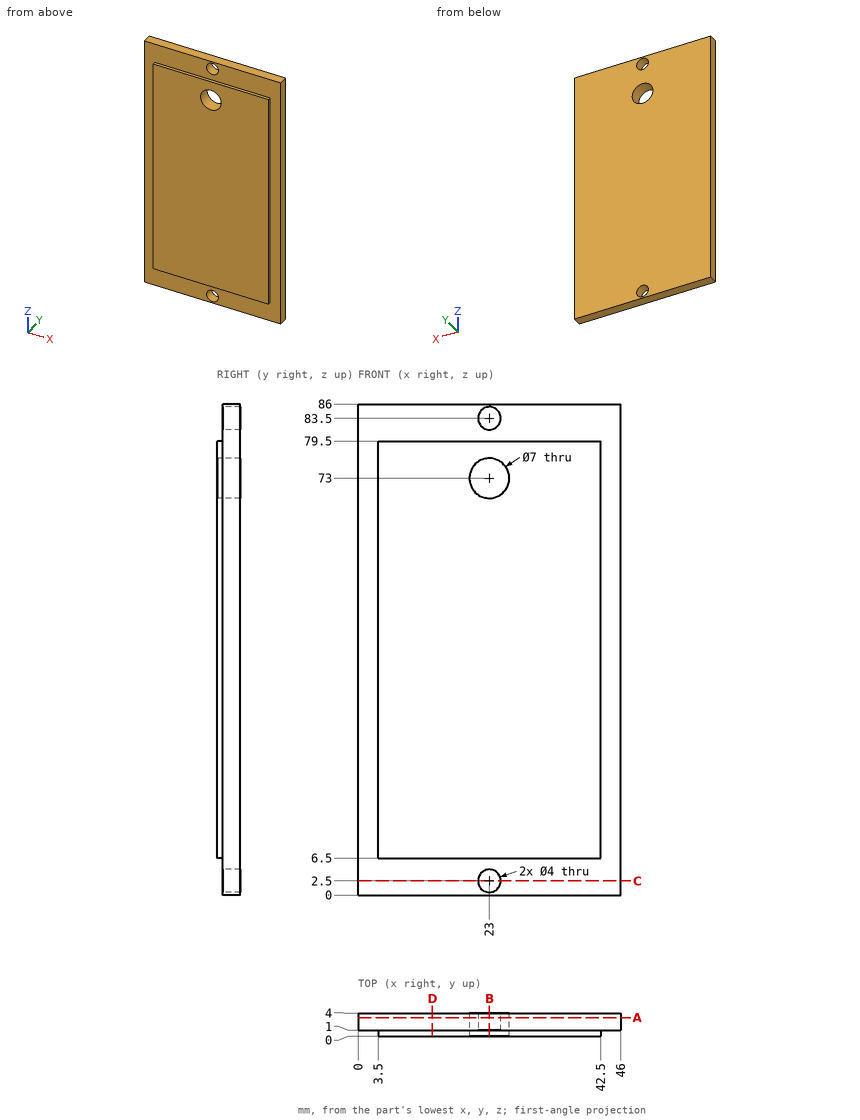
Job drawing, mm, ordinate dimensions from the low corner. One solid piece. Coordinates: 2 decimals unless noted, no trailing zeros. Order: outer loops, then holes, each group sorted by start corner. A loop starts at its lowest first (then second) coordinate and runs counter-clockwise, first axis right, second up. Notation, with made-up numbers: M 33,62 L 87,62 A30 ccw 87,86 Z; hole C 71.25,-30.5 d1. An arc over 180 degrees is marked long. Return JSON: item names as keys, results as strings.
1. Drill centre lines: probe 1 along Z at (x, y) = (23, 2.3); probe 2 along X at (y, z) = (2.5, 83.5); probe 3 along Z at (x, y) = (24.5, 3.1). Where is each one in solid material? Low to high.
Ans:
{"probe 1": "0 to 0.5, 4.5 to 69.5, 76.5 to 81.5, 85.5 to 86", "probe 2": "0 to 21, 25 to 46", "probe 3": "0 to 1.18, 3.82 to 69.84, 76.16 to 82.18, 84.82 to 86"}
2. Saw through at A-A (y = 3.2). Give the cut face in (x, z).
Ans:
{"outline": "M 0,0 L 46,0 L 46,86 L 0,86 Z; hole C 23,73 d7; hole C 23,2.5 d4; hole C 23,83.5 d4"}
3. Flat gauge pins, fed straight in: pin 1 (23 mm diameter, centred on x = 13.5, z = 45.5, fed in from -Y); pin 2 (0.5 mm diameter, centred on x = 20.5, y = 0.5, fed in from -Z); pin 3 (0.5 mm diameter, centred on x = 15, y = 0.5, fed in from +Z). Where does each tip first touch, or does it go through?
Ans:
{"pin 1": "y = 0", "pin 2": "z = 6.5", "pin 3": "z = 79.5"}
4. Saw through at D-D (x = 13). Give the cut face in (y, z), and give its area (3 significant figures).
Ans:
{"outline": "M 0,6.5 L 1,6.5 L 1,0 L 4,0 L 4,86 L 1,86 L 1,79.5 L 0,79.5 Z", "area": "331 mm^2"}
5. Saw through at B-B (x = 23). Give the cut face in (y, z), and give its area (3 significant figures).
Ans:
{"outline": "M 0,6.5 L 1,6.5 L 1,4.5 L 4,4.5 L 4,69.5 L 0,69.5 Z; M 0,76.5 L 4,76.5 L 4,81.5 L 1,81.5 L 1,79.5 L 0,79.5 Z; M 1,0 L 4,0 L 4,0.5 L 1,0.5 Z; M 1,85.5 L 4,85.5 L 4,86 L 1,86 Z", "area": "279 mm^2"}
6. Saw through at C-C (z = 2.5). Give the cut face in (x, y), and give its area (3 significant figures).
Ans:
{"outline": "M 0,1 L 21,1 L 21,4 L 0,4 Z; M 25,1 L 46,1 L 46,4 L 25,4 Z", "area": "126 mm^2"}
